from build123d import *

# Parameters (mm, degrees)
SKETCH1_R           = 21.4
BOSS_EXTRUDE1_DEPTH = 68
SKETCH2_W           = 60
SKETCH2_H           = 60
SKETCH2_R           = 2
BOSS_EXTRUDE2_DEPTH = 31.3
SKETCH3_R           = 12.5
BOSS_EXTRUDE3_DEPTH = 2
FILLET1_R           = 3
SKETCH4_R           = 4
BOSS_EXTRUDE4_DEPTH = 8
BOSS_EXTRUDE5_DEPTH = 18
FILLET2_R           = 3
BOSS_EXTRUDE6_DEPTH = 7
CUT_EXTRUDE1_REACH  = 141.197
SKETCH7_R           = 1.686317599


with BuildPart() as part:
    # Sketch1 → Boss-Extrude1 (new body)
    with BuildSketch(Plane.XY):
        Circle(SKETCH1_R)
    extrude(amount=BOSS_EXTRUDE1_DEPTH)

    # Sketch2 → Boss-Extrude2 (add)
    with BuildSketch(Plane.XY.offset(68)):
        Rectangle(SKETCH2_W, SKETCH2_H)
        with Locations((-24.75, 24.75)):
            Circle(SKETCH2_R, mode=Mode.SUBTRACT)
        with Locations((24.75, 24.75)):
            Circle(SKETCH2_R, mode=Mode.SUBTRACT)
        with Locations(Location((24.75, -24.75, 0), (0, 0, 180))):
            Circle(SKETCH2_R, mode=Mode.SUBTRACT)
        with Locations(Location((-24.75, -24.75, 0), (0, 0, 180))):
            Circle(SKETCH2_R, mode=Mode.SUBTRACT)
    extrude(amount=BOSS_EXTRUDE2_DEPTH)

    # Sketch3 → Boss-Extrude3 (add)
    with BuildSketch(Plane.XY.offset(99.3)):
        with Locations((0, -10)):
            Circle(SKETCH3_R)
    extrude(amount=BOSS_EXTRUDE3_DEPTH)

    # Fillet1
    # the kernel refuses this fillet: 3 mm, written as the material it takes off along each edge
    with BuildSketch(Plane(origin=(0, -10, 101.3), x_dir=(1, 0, 0), z_dir=(0, -1, 0))) as fillet1_piece_1:
        with BuildLine():
            CenterArc((9.671572875, -3), FILLET1_R, 19.471220634, 70.528779366)
            Line((9.671572875, 0), (9.671572875, 0.06))
            Line((9.671572875, 0.06), (12.5, 0.06))
            Line((12.5, 0.06), (12.56, 0))
            ThreePointArc((12.56, 0), (12.56, -1), (12.556568542, -1.98))
            Line((12.556568542, -1.98), (12.5, -2))
        make_face()
    revolve(axis=Axis((0, -10, 101.3), (0, 0, 1)), mode=Mode.SUBTRACT)

    # Sketch4 → Boss-Extrude4 (add)
    with BuildSketch(Plane.XY.offset(101.3)):
        with Locations((0, -10)):
            Circle(SKETCH4_R)
    extrude(amount=BOSS_EXTRUDE4_DEPTH)

    # Sketch5 → Boss-Extrude5 (add)
    with BuildSketch(Plane.XY.offset(109.3)):
        with BuildLine():
            Line((1.936491673, -6.5), (-1.936491673, -6.5))
            ThreePointArc((-1.936491673, -6.5), (-2.031506006, -13.445719569), (4, -10))
            ThreePointArc((4, -10), (3.445719569, -7.968493994), (1.936491673, -6.5))
        make_face()
    extrude(amount=BOSS_EXTRUDE5_DEPTH)

    # Fillet2
    fillet2_edges = [part.edges().sort_by_distance(p)[0] for p in [
        (-30, -30, 83.65),
        (30, -30, 83.65),
        (30, 30, 83.65),
        (-30, 30, 83.65),
    ]]
    fillet(fillet2_edges, radius=FILLET2_R)

    # Sketch6 → Boss-Extrude6 (add)
    with BuildSketch(Plane(origin=(0, 0, 0), x_dir=(-1, 0, 0), z_dir=(0, 0, -1))):
        with BuildLine():
            Line((-2.5, 17.65), (2.5, 17.65))
            ThreePointArc((2.5, 17.65), (3, 17.15), (2.5, 16.65))
            Line((2.5, 16.65), (-2.5, 16.65))
            ThreePointArc((-2.5, 16.65), (-3, 17.15), (-2.5, 17.65))
        make_face()
        with BuildLine():
            Line((-2.5, -17.65), (2.5, -17.65))
            ThreePointArc((2.5, -17.65), (3, -17.15), (2.5, -16.65))
            Line((2.5, -16.65), (-2.5, -16.65))
            ThreePointArc((-2.5, -16.65), (-3, -17.15), (-2.5, -17.65))
        make_face()
    extrude(amount=BOSS_EXTRUDE6_DEPTH)

    # Cut-Extrude1: up to this face of the body (flat: up to its plane)
    cut_extrude1_end = Plane(part.part.faces().sort_by_distance((0, -17.65, -3.5))[0])
    # Sketch7 → Cut-Extrude1 (cut, up to the picked face)
    with BuildSketch(Plane(origin=(0, 17.65, 0), x_dir=(1, 0, 0), z_dir=(0, 1, 0)), mode=Mode.PRIVATE) as cut_extrude1_sk1:
        with Locations(Location((0, 4.176322203, 0), (0, 0, 270))):
            Circle(SKETCH7_R)
    cut_extrude1_tool1 = split(extrude(cut_extrude1_sk1.sketch, amount=-CUT_EXTRUDE1_REACH, mode=Mode.PRIVATE), bisect_by=cut_extrude1_end, keep=Keep.BOTH, mode=Mode.PRIVATE)
    add(cut_extrude1_tool1.solids().sort_by(Axis((0, 17.65, -4.176322), (0, -1, 0)))[0], mode=Mode.SUBTRACT)


solid = part.part
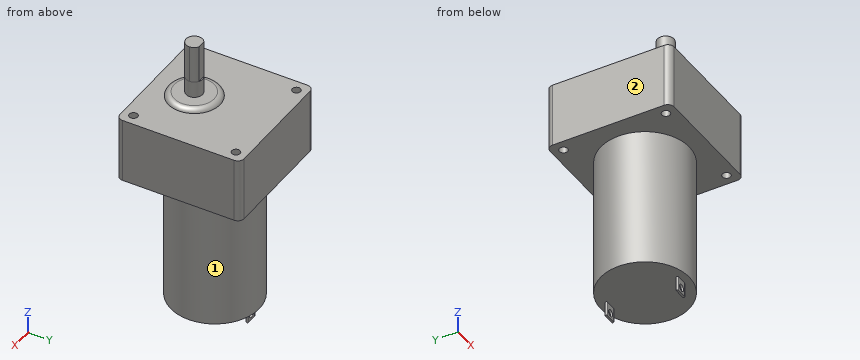
Geometry check sheet. Reference: the model listing, model coordinates, mm. Face numbers are marked on the shaded views. A direction names the side the tool comes from. Coordinates: 2 decimals unless noted, no trailing zeros. Loops run counter-clockwise (first coordinate to the right, second up) from the corner with the lowest first, then second, coordinate; pieces in that order, holes last. Notation, with made-up numbers: (51, -17) - (77, -17) arc R31 ccw to (77, 18) - close; hole circle Ø11 at (-10, 42.25). An arc over 180 degrees is marked (long way). Use one line per item in the form item = value. Start each with the question number.
Item 1: Section check B-B, the plane z = 87.5. Enter the section's corners in (x, y).
Item 2: Tool access check on the marked faces 1 and 2. Record the directions out of +Z, -Z, +X, -X, +Y, -Y that give a thin tool (end or side, any length) a straight path to the whole face; none if there is none.
Item 3: Thickness scan on probe 1 along Y at (x, z) = (24.75, 80); probe 2 along X at (y, z) = (-24, 84). Record the ranges inside material, lowest first.
Item 4: Section check A-A, the plane x = -24.75. Enter the section's corners in (y, z).
Item 5: Gauge pin test, flat ends, axial feed: pin 1 (1.5 mm diameter, centred on x = -0.5, z = -2.5, fed in from -Y); pin 2 (3 mm diameter, centred on x = 0, z = -4.18, fed in from -Y); pin 3 (5 mm diameter, centred on x = -24.75, y = -24.75, fed in from -Z); pin 4 (2 mm diameter, centred on x = -2.5, z = 34, fed in from +Y). Record the tip position at first contact, or that the pin passes through.
Item 6: Section check D-D, the plane y = 6. Enter the section's corners in (x, z), and give its area (3 significant figures).
Computed:
q1.outline = (-30, -27) arc R3 ccw to (-27, -30) - (27, -30) arc R3 ccw to (30, -27) - (30, 27) arc R3 ccw to (27, 30) - (-27, 30) arc R3 ccw to (-30, 27) - close; hole circle Ø4 at (-24.75, -24.75); hole circle Ø4 at (-24.75, 24.75); hole circle Ø4 at (24.75, -24.75); hole circle Ø4 at (24.75, 24.75)
q2.face_1 = -Z
q2.face_2 = +Z, -Z, -X, +Y, -Y
q3.probe_1 = -30 to -26.75, -22.75 to 22.75, 26.75 to 30
q3.probe_2 = -30 to -26.6, -22.9 to 22.9, 26.6 to 30
q4.outline = (-30, 68) - (-26.75, 68) - (-26.75, 99.3) - (-30, 99.3) - close; (-22.75, 68) - (22.75, 68) - (22.75, 99.3) - (-22.75, 99.3) - close; (26.75, 68) - (30, 68) - (30, 99.3) - (26.75, 99.3) - close
q5.pin_1 = -17.65
q5.pin_2 = through
q5.pin_3 = 68
q5.pin_4 = 21.35
q6.outline = (-30, 68) - (-20.54, 68) - (-20.54, 0) - (20.54, 0) - (20.54, 68) - (30, 68) - (30, 99.3) - (-30, 99.3) - close
q6.area = 4,670 mm2
